Could you check a few things on this model? Use its own coordinates, in mm. Give positions to 0.01 mm unless a question says otherwise; leave off trailing zeros. Loops run counter-clockwise (first coordinate to the right, second up) from the corner with the lowest first, then second, coordinate; pieces in that order, holes last. Notation, with made-up numbers: M 80,-16.75 L 116,-16.75 A34 cw 116,21.25 Z; hole C 60,18.5 d5. An arc over 180 degrees is marked long. Return JSON: item names as keys, results as strings. Group by question number.
1. If we mould it in two halves opening along X, with no side actions, what happens to faces 1 (the flat face through (203, 3, -102)), 2 (the cylindrical face through (104.06, 1.48, -164.42)), 3 (the cylindrical face through (242.68, 1.48, -101.63))? For each: +X half, -X half, draft (parallel to the pull), parting line (faces both ways), or undercut.
2. Please list where these lines run through material, in increasing order: line 1 (X direction, y = 2.4, z = -210); line 2 (X direction, y = 1.15, z = -161); line 3 (Z direction, x = 108, y = 1.25).
3. If we section it at A-A (z = -160): Write out the boundary of the cut face in (x, y).
```python
from build123d import *

# Parameters (mm, degrees)
SKETCH_1_R      = 5.1
SKETCH_1_R_2    = 1.5
SKETCH_1_R_3    = 7.5
SKETCH_1_R_4    = 6
SKETCH_1_R_5    = 1.7
SKETCH_1_R_6    = 2.5
EXTRUDE_1_DEPTH = 3


with BuildPart() as part:
    # 草图1 → 凸台-拉伸1 (new body)
    with BuildSketch(Plane(origin=(0, 0, 0), x_dir=(1, 0, 0), z_dir=(0, 1, 0))):
        with BuildLine():
            Line((-23, 220), (423, 220))
            ThreePointArc((423, 220), (424.414213562, 219.414213562), (425, 218))
            Line((425, 218), (425, -18))
            ThreePointArc((425, -18), (424.414213562, -19.414213562), (423, -20))
            Line((423, -20), (-23, -20))
            ThreePointArc((-23, -20), (-24.414213562, -19.414213562), (-25, -18))
            Line((-25, -18), (-25, 218))
            ThreePointArc((-25, 218), (-24.414213562, 219.414213562), (-23, 220))
        make_face()
        with Locations(Location((100, 100, 0), (0, 0, 270))):
            Circle(SKETCH_1_R, mode=Mode.SUBTRACT)
        with Locations(Location((150, 112, 0), (0, 0, 270))):
            Circle(SKETCH_1_R_2, mode=Mode.SUBTRACT)
        with Locations(Location((100, 92, 0), (0, 0, 270))):
            Circle(SKETCH_1_R_2, mode=Mode.SUBTRACT)
        with Locations(Location((108, 100, 0), (0, 0, 270))):
            Circle(SKETCH_1_R_2, mode=Mode.SUBTRACT)
        with Locations(Location((92, 100, 0), (0, 0, 270))):
            Circle(SKETCH_1_R_2, mode=Mode.SUBTRACT)
        with Locations(Location((100, 108, 0), (0, 0, 270))):
            Circle(SKETCH_1_R_2, mode=Mode.SUBTRACT)
        with Locations(Location((50, 100, 0), (0, 0, 270))):
            Circle(SKETCH_1_R_3, mode=Mode.SUBTRACT)
        with Locations(Location((50, 112, 0), (0, 0, 270))):
            Circle(SKETCH_1_R_2, mode=Mode.SUBTRACT)
        with Locations(Location((62, 100, 0), (0, 0, 270))):
            Circle(SKETCH_1_R_2, mode=Mode.SUBTRACT)
        with Locations(Location((50, 88, 0), (0, 0, 270))):
            Circle(SKETCH_1_R_2, mode=Mode.SUBTRACT)
        with Locations(Location((38, 100, 0), (0, 0, 270))):
            Circle(SKETCH_1_R_2, mode=Mode.SUBTRACT)
        with Locations(Location((162, 100, 0), (0, 0, 270))):
            Circle(SKETCH_1_R_2, mode=Mode.SUBTRACT)
        with Locations(Location((138, 100, 0), (0, 0, 270))):
            Circle(SKETCH_1_R_2, mode=Mode.SUBTRACT)
        with Locations(Location((150, 88, 0), (0, 0, 270))):
            Circle(SKETCH_1_R_2, mode=Mode.SUBTRACT)
        with Locations(Location((150, 100, 0), (0, 0, 270))):
            Circle(SKETCH_1_R_3, mode=Mode.SUBTRACT)
        with Locations(Location((100, 160, 0), (0, 0, 270))):
            Circle(SKETCH_1_R_4, mode=Mode.SUBTRACT)
        with Locations(Location((300, 100, 0), (0, 0, 270))):
            Circle(SKETCH_1_R, mode=Mode.SUBTRACT)
        with Locations(Location((350, 112, 0), (0, 0, 270))):
            Circle(SKETCH_1_R_2, mode=Mode.SUBTRACT)
        with Locations(Location((300, 108, 0), (0, 0, 270))):
            Circle(SKETCH_1_R_2, mode=Mode.SUBTRACT)
        with Locations(Location((308, 100, 0), (0, 0, 270))):
            Circle(SKETCH_1_R_2, mode=Mode.SUBTRACT)
        with Locations(Location((300, 92, 0), (0, 0, 270))):
            Circle(SKETCH_1_R_2, mode=Mode.SUBTRACT)
        with Locations(Location((292, 100, 0), (0, 0, 270))):
            Circle(SKETCH_1_R_2, mode=Mode.SUBTRACT)
        with Locations(Location((250, 100, 0), (0, 0, 270))):
            Circle(SKETCH_1_R_3, mode=Mode.SUBTRACT)
        with Locations(Location((250, 112, 0), (0, 0, 270))):
            Circle(SKETCH_1_R_5, mode=Mode.SUBTRACT)
        with Locations(Location((262, 100, 0), (0, 0, 270))):
            Circle(SKETCH_1_R_2, mode=Mode.SUBTRACT)
        with Locations(Location((250, 88, 0), (0, 0, 270))):
            Circle(SKETCH_1_R_2, mode=Mode.SUBTRACT)
        with Locations(Location((238, 100, 0), (0, 0, 270))):
            Circle(SKETCH_1_R_2, mode=Mode.SUBTRACT)
        with Locations(Location((362, 100, 0), (0, 0, 270))):
            Circle(SKETCH_1_R_2, mode=Mode.SUBTRACT)
        with Locations(Location((338, 100, 0), (0, 0, 270))):
            Circle(SKETCH_1_R_2, mode=Mode.SUBTRACT)
        with Locations(Location((350, 88, 0), (0, 0, 270))):
            Circle(SKETCH_1_R_2, mode=Mode.SUBTRACT)
        with Locations(Location((350, 100, 0), (0, 0, 270))):
            Circle(SKETCH_1_R_3, mode=Mode.SUBTRACT)
        with Locations(Location((300, 160, 0), (0, 0, 270))):
            Circle(SKETCH_1_R_4, mode=Mode.SUBTRACT)
        with Locations(Location((415, -10, 0), (0, 0, 270))):
            Circle(SKETCH_1_R_6, mode=Mode.SUBTRACT)
        with Locations(Location((100, -10, 0), (0, 0, 270))):
            Circle(SKETCH_1_R_6, mode=Mode.SUBTRACT)
        with Locations(Location((300, -10, 0), (0, 0, 270))):
            Circle(SKETCH_1_R_6, mode=Mode.SUBTRACT)
        with Locations(Location((-15, -10, 0), (0, 0, 270))):
            Circle(SKETCH_1_R_6, mode=Mode.SUBTRACT)
        with Locations(Location((200, -10, 0), (0, 0, 270))):
            Circle(SKETCH_1_R_6, mode=Mode.SUBTRACT)
        with Locations(Location((200, 210, 0), (0, 0, 270))):
            Circle(SKETCH_1_R_6, mode=Mode.SUBTRACT)
        with Locations(Location((-15, 210, 0), (0, 0, 270))):
            Circle(SKETCH_1_R_6, mode=Mode.SUBTRACT)
        with Locations(Location((300, 210, 0), (0, 0, 270))):
            Circle(SKETCH_1_R_6, mode=Mode.SUBTRACT)
        with Locations(Location((100, 210, 0), (0, 0, 270))):
            Circle(SKETCH_1_R_6, mode=Mode.SUBTRACT)
        with Locations(Location((415, 210, 0), (0, 0, 270))):
            Circle(SKETCH_1_R_6, mode=Mode.SUBTRACT)
    extrude(amount=EXTRUDE_1_DEPTH)


solid = part.part
```
Answer:
{
 "1": {"face 1": "draft", "face 2": "undercut", "face 3": "undercut"},
 "2": {"line 1": "x = -25 to -17.5, -12.5 to 97.5, 102.5 to 197.5, 202.5 to 297.5, 302.5 to 412.5, 417.5 to 425", "line 2": "x = -25 to 94.08, 105.92 to 294.08, 305.92 to 425", "line 3": "z = -220 to -101.5, -98.5 to 20"},
 "3": {"outline": "M -25,0 L 94,0 L 94,3 L -25,3 Z; M 106,0 L 294,0 L 294,3 L 106,3 Z; M 306,0 L 425,0 L 425,3 L 306,3 Z"}
}
